Answer from the drawing. Dimensions are ordinates in mm from the lowest x, y and z of the part. A direction names the side the tool comes from. Round coordinates to 2 decimals unless told otherwise and drop trailing zeros. Loops run counter-clockwise (first coordinate to the right, second up) from the corner with the lowest first, then second, coordinate; pieces in that order, holes last. Notation, with made-up numbers: (42, -16) - (79, -16) arc R14 cw to (79, 10) - close; hole circle Ø11 at (4.5, 3). An arc over 180 degrees is marked (long way). Write item = value, one per line. Start each with the question number.
1) Straight lines are drawn through the part: line 1 along X through (y, z) = (9.5, 4.5); line 2 along X through (y, z) = (8.5, 12.5); line 3 along Y through (x, z) = (43, 9.75). For each, find the intervals that lie inside material, in ascending order.
2) Given pin 1 Ø10 at (y, z) = (3, 12.5) entering from +X; pin 2 Ø12 at (x, z) = (45.5, 5) entering from -Y; pin 3 Ø1.5 at (x, z) = (38.5, 2) entering from -Y; pin 4 Ø10 at (x, y) = (39, 4) entering from +Z, each flat-ended and moving along its own axis, determine where each tip first touches the part or whether it passes through.
3) A tool of negligible diameter and unlimited length cuts with its end or side. For the marked faces 1, 2 and 3, from which of +Z, -Z, +X, -X, +Y, -Y can it reach the whole face along a straight path? Write none if from no direction.
4) Section C-C, the plane x = 5 is taken. Determine the outline of the cut face in (y, z).
5) Section A-A, the plane z = 10 is taken. Determine the outline of the cut face in (x, y).
6) Section B-B, the plane x = 43.5 is taken. Determine the outline of the cut face in (y, z).
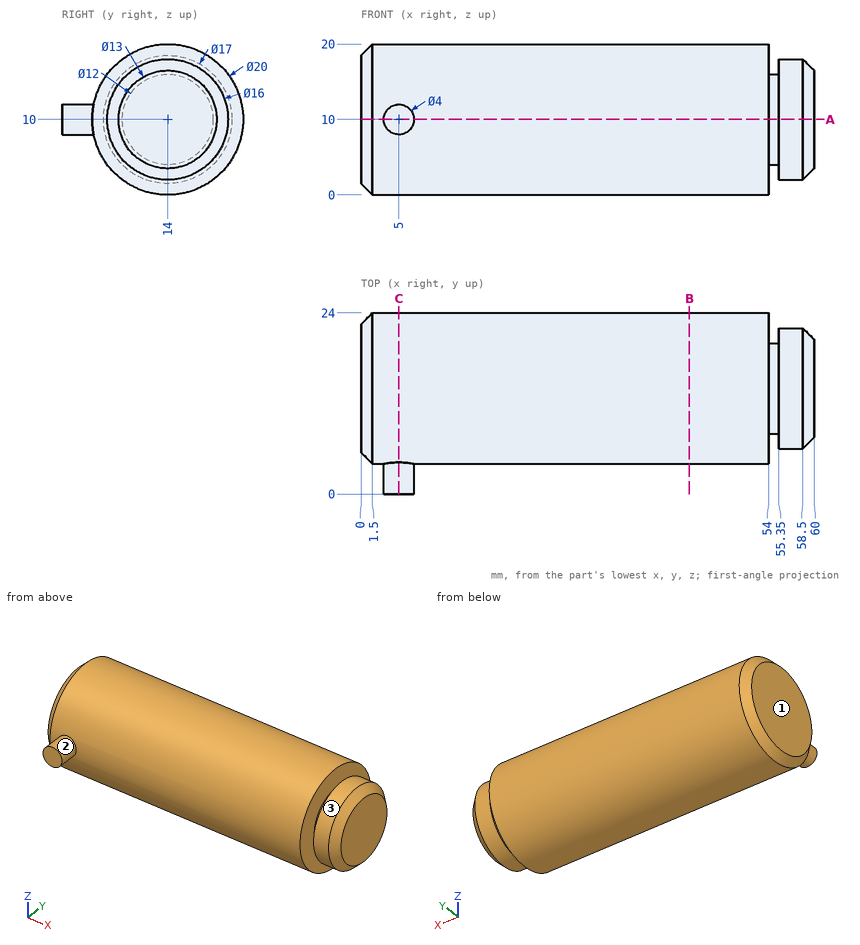
Geometry check:
q1.line_1 = 0 to 54, 55.35 to 59.39
q1.line_2 = 0 to 54, 55.35 to 60
q1.line_3 = 4 to 24
q2.pin_1 = 60
q2.pin_2 = 4
q2.pin_3 = 7.11
q2.pin_4 = 18.66
q3.face_1 = +Z, -Z, -X, +Y, -Y
q3.face_2 = -Y
q3.face_3 = +X
q4.outline = (0, 8) - (4.2, 8) arc R10 ccw (long way) to (4.2, 12) - (0, 12) - close
q5.outline = (0, 5.5) - (1.5, 4) - (3, 4) - (3, 0) - (7, 0) - (7, 4) - (54, 4) - (54, 8) - (55.35, 8) - (55.35, 6) - (58.5, 6) - (60, 7.5) - (60, 20.5) - (58.5, 22) - (55.35, 22) - (55.35, 20) - (54, 20) - (54, 24) - (1.5, 24) - (0, 22.5) - close
q6.outline = circle Ø20 at (14, 10)
